Read the model definition and answer for the solid it produces. Units are mm, in the model's axes. A direction names the side the tool comes from. Coordinates: 2 decimals unless noted, no trailing zeros. Write each loop counter-clockwise with the first axis right and the second up, starting at its lowest first coordinate (ties: lowest second). Pieces come first, ordered by that corner, then holes. Notation, with made-up numbers: (-11.75, 84.5) -> (24.25, 84.5) arc R23 ccw to (24.25, 93.5) -> close; hole circle Ø3 at (10.25, 24). An arc over 180 degrees is marked (long way). Write item = value, one per line. Start each with the question number.
1) Find the intervals of material crossed by line 1 along X through (y, z) = (-10, 20.75); line 2 along Y through (x, z) = (0, 19.3); line 3 along X through (y, z) = (-17, 18), in increasing order. Write a range as from..to.
2) For a pull along X with two mould halves and no side action, classify faces 1 (the face through (-9.92, -9.459, 22.084)), 2 (the face through (4.68, -9.46, 23.49)), 3 (the face through (6.666, -9.459, 19.622)) as released by +X, released by -X, zero draft, split by the parting line, or undercut.
3) A tool of negligible diameter and unlimited length cuts with its end or side. For faces 4 (the face through (-4.57, -9.73, 22.14)), 5 (the face through (-3.293, -9.459, 23.985)), 6 (the face through (-1.588, -10, 23)), from which of +Z, -Z, +X, -X, +Y, -Y can it reach the whole face along a straight path? Write none if from no direction.
4) Section A-A (z = 17) is taken. Determine the outline of the cut face in (x, y), plus the area to 3 significant figures.
5) Section B-B (y = -5.5) is taken. Count the separate pieces of the cut face and the enclosed holes in it, plus the area to 3 significant figures.
6) Flat-ended cylindrical pins translate along their axes: pin 1 Ø1.6 at (x, z) = (9.52, 18.75) entering from +Y; pin 2 Ø0.7 at (y, z) = (-7.5, 23) entering from -X; pin 3 Ø4 at (y, z) = (-12, 16.5) entering from +X; pin 4 Ø1 at (x, y) = (3.5, -14) entering from -Z. Find the tip coordinate at first contact, or state that the pin passes through.
from build123d import *

# Parameters (mm, degrees)
F0_R     = 1.35255
F1_DEPTH = 19.18716
F2_W     = 3.175
F2_H     = 3.96875
F3_DEPTH = 19.18716
F4_R     = 1.58749
F5_R     = 0.79375
F6_R     = 0.79375
F7_DEPTH = 55


# Not quite as in the source:
# - a fillet or chamfer is up to 0.001 mm smaller than in the source, because OpenCascade refuses the exact size
# - an extrude ends at something that could not be found from the text; its depth is read off the source's solid


with BuildPart() as f1:
    # F0 (on Front) → F1 (new body)
    with BuildSketch(Plane.XZ):
        with BuildLine():
            ThreePointArc((-8.0873006088, 15.9239409983), (0, 17.8599084), (8.0873006088, 15.9239409983))
            ThreePointArc((8.0873006088, 15.9239409983), (12.3558382964, 17.3170799036), (10.9626993912, 21.5856175912))
            ThreePointArc((10.9626993912, 21.5856175912), (0, 24.2099084), (-10.9626993912, 21.5856175912))
            ThreePointArc((-10.9626993912, 21.5856175912), (-12.3558382964, 17.3170799036), (-8.0873006088, 15.9239409983))
        make_face()
        with Locations((-9.525, 18.7547792948)):
            Circle(F0_R, mode=Mode.SUBTRACT)
        with Locations((9.525, 18.7547792948)):
            Circle(F0_R, mode=Mode.SUBTRACT)
    extrude(amount=F1_DEPTH)

    # F2 (on face) → F3 (cut, through all)
    with BuildSketch(Plane.XZ.offset(19.18716)):
        Polygon((-8.0765705738, 22.8781299226), (-7.0031118134, 19.0573102654), (-3.9464560877, 19.9160772737), (-5.0199148481, 23.7368969308), align=None)
        Polygon((8.0765705738, 22.8781299226), (5.0199148481, 23.7368969308), (3.9464560877, 19.9160772737), (7.0031118134, 19.0573102654), align=None)
        with Locations((0, 22.2255334)):
            Rectangle(F2_W, F2_H)
    extrude(amount=-F3_DEPTH, mode=Mode.SUBTRACT)

    # F4 (radius 1.5875 in the source; OpenCascade refuses exactly that, so slightly less here)
    f4_edges = [f1.edges().sort_by_distance(p)[0] for p in [
        (-7.003112, -9.59358, 19.05731),
        (-3.946456, -9.59358, 19.916077),
        (-1.5875, -9.59358, 20.241158),
        (1.5875, -9.59358, 20.241158),
        (3.946456, -9.59358, 19.916077),
        (7.003112, -9.59358, 19.05731),
    ]]
    fillet(f4_edges, radius=F4_R)

    # F5
    f5_edges = [f1.edges().sort_by_distance(p)[0] for p in [
        (-8.062478, -9.59358, 22.827968),
        (-5.005822, -9.59358, 23.686735),
        (-1.5875, -9.59358, 24.157804),
        (1.5875, -9.59358, 24.157804),
        (5.005822, -9.59358, 23.686735),
        (8.062478, -9.59358, 22.827968),
    ]]
    fillet(f5_edges, radius=F5_R)

    # F6 (on Top) → F7 (cut, through all)
    with BuildSketch(Plane.XY):
        with Locations((0, -9.59358)):
            Circle(F6_R)
    extrude(amount=F7_DEPTH, mode=Mode.SUBTRACT)


solid = f1.part
Answer key:
q1.line_1 = -11.99..-7.48, -4.34..-1.16, 1.16..4.34, 7.48..11.99
q1.line_2 = -19.19..-10.39, -8.8..0
q1.line_3 = -12.61..-10.65, -8.4..8.4, 10.65..12.61
q2.face_1 = released by -X
q2.face_2 = released by +X
q2.face_3 = undercut
q3.face_4 = +Y, -Y
q3.face_5 = +Z, -X, +Y, -Y
q3.face_6 = +Z, +Y, -Y
q4.outline = (-12.17, -19.19) -> (-5.48, -19.19) -> (-5.48, 0) -> (-12.17, 0) -> close; (5.48, -19.19) -> (12.17, -19.19) -> (12.17, 0) -> (5.48, 0) -> close
q4.area = 257 mm^2
q5.separate_pieces = 1
q5.enclosed_holes = 2
q5.area = 110 mm^2
q6.pin_1 = through
q6.pin_2 = -4.8
q6.pin_3 = 12.69
q6.pin_4 = 17.41
